from build123d import *

# Parameters (mm, degrees)
SKETCH1_W           = 100
SKETCH1_H           = 48
BOSS_EXTRUDE1_DEPTH = 7
CUT_EXTRUDE1_REACH  = 113.144
SKETCH2_R           = 4
SKETCH2_R_2         = 3.5
SKETCH3_W           = 100
SKETCH3_H           = 8
BOSS_EXTRUDE2_DEPTH = 10.2
SKETCH4_R           = 6.55
CUT_EXTRUDE2_DEPTH  = 5.25
SKETCH5_R           = 2.6
CUT_EXTRUDE3_DEPTH  = 7
SKETCH7_R           = 1.7
CUT_EXTRUDE4_DEPTH  = 112.391382072
CUT_EXTRUDE5_REACH  = 114.249
SKETCH8_R           = 1.7
CUT_EXTRUDE6_DEPTH  = 3
CUT_EXTRUDE7_REACH  = 114.249
SKETCH10_R          = 1.7
CUT_EXTRUDE8_DEPTH  = 3
FILLET1_R           = 20


with BuildPart() as part:
    # Sketch1 → Boss-Extrude1 (new body)
    with BuildSketch(Plane.XY):
        with Locations((50, 24)):
            Rectangle(SKETCH1_W, SKETCH1_H)
    extrude(amount=BOSS_EXTRUDE1_DEPTH)

    # Sketch2 → Cut-Extrude1 (cut, up to next)
    with BuildSketch(Plane.XY.offset(7), mode=Mode.PRIVATE) as cut_extrude1_sk1:
        with BuildLine():
            ThreePointArc((15, 25), (11, 29), (15, 33))
            Line((15, 33), (0, 33))
            Line((0, 33), (0, 25))
            Line((0, 25), (15, 25))
        make_face()
    cut_extrude1_tool1 = extrude(cut_extrude1_sk1.sketch, amount=-CUT_EXTRUDE1_REACH, mode=Mode.PRIVATE) & part.part
    # Sketch2 → Cut-Extrude1 (cut, up to next)
    with BuildSketch(Plane.XY.offset(7), mode=Mode.PRIVATE) as cut_extrude1_sk2:
        with Locations((15, 29)):
            Circle(SKETCH2_R)
    cut_extrude1_tool2 = extrude(cut_extrude1_sk2.sketch, amount=-CUT_EXTRUDE1_REACH, mode=Mode.PRIVATE) & part.part
    # Sketch2 → Cut-Extrude1 (cut, up to next)
    with BuildSketch(Plane.XY.offset(7), mode=Mode.PRIVATE) as cut_extrude1_sk3:
        with Locations((33.75, 29)):
            Circle(SKETCH2_R_2)
    cut_extrude1_tool3 = extrude(cut_extrude1_sk3.sketch, amount=-CUT_EXTRUDE1_REACH, mode=Mode.PRIVATE) & part.part
    # Sketch2 → Cut-Extrude1 (cut, up to next)
    with BuildSketch(Plane.XY.offset(7), mode=Mode.PRIVATE) as cut_extrude1_sk4:
        with Locations((55, 29)):
            Circle(SKETCH2_R_2)
    cut_extrude1_tool4 = extrude(cut_extrude1_sk4.sketch, amount=-CUT_EXTRUDE1_REACH, mode=Mode.PRIVATE) & part.part
    # Sketch2 → Cut-Extrude1 (cut, up to next)
    with BuildSketch(Plane.XY.offset(7), mode=Mode.PRIVATE) as cut_extrude1_sk5:
        with Locations((76.25, 29)):
            Circle(SKETCH2_R_2)
    cut_extrude1_tool5 = extrude(cut_extrude1_sk5.sketch, amount=-CUT_EXTRUDE1_REACH, mode=Mode.PRIVATE) & part.part
    add(cut_extrude1_tool1.solids().sort_by_distance((5.962811, 29, 7))[0], mode=Mode.SUBTRACT)
    add(cut_extrude1_tool2.solids().sort_by_distance((15, 29, 7))[0], mode=Mode.SUBTRACT)
    add(cut_extrude1_tool3.solids().sort_by_distance((33.75, 29, 7))[0], mode=Mode.SUBTRACT)
    add(cut_extrude1_tool4.solids().sort_by_distance((55, 29, 7))[0], mode=Mode.SUBTRACT)
    add(cut_extrude1_tool5.solids().sort_by_distance((76.25, 29, 7))[0], mode=Mode.SUBTRACT)

    # Sketch3 → Boss-Extrude2 (add)
    with BuildSketch(Plane(origin=(0, 0, 0), x_dir=(-1, 0, 0), z_dir=(0, 0, -1))):
        with Locations((-50, 4)):
            Rectangle(SKETCH3_W, SKETCH3_H)
    extrude(amount=BOSS_EXTRUDE2_DEPTH)

    # Sketch4 → Cut-Extrude2 (cut)
    with BuildSketch(Plane(origin=(0, 0, 0), x_dir=(-1, 0, 0), z_dir=(0, 0, -1))):
        with Locations((-76.25, 29)):
            Circle(SKETCH4_R)
        with Locations((-55, 29)):
            Circle(SKETCH4_R)
        with Locations((-33.75, 29)):
            Circle(SKETCH4_R)
    extrude(amount=-CUT_EXTRUDE2_DEPTH, mode=Mode.SUBTRACT)

    # Sketch5 → Cut-Extrude3 (cut)
    with BuildSketch(Plane.XY.offset(7)):
        with Locations((35.000022648, 4.052132501)):
            Circle(SKETCH5_R)
        with Locations((64.999977352, 4)):
            Circle(SKETCH5_R)
    extrude(amount=-CUT_EXTRUDE3_DEPTH, mode=Mode.SUBTRACT)

    # Sketch7 → Cut-Extrude4 (cut, through all)
    with BuildSketch(Plane.XY):
        with Locations((35.000022648, 4.052132501)):
            Circle(SKETCH7_R)
        with Locations((64.999977352, 4)):
            Circle(SKETCH7_R)
    extrude(amount=-CUT_EXTRUDE4_DEPTH, mode=Mode.SUBTRACT)

    # Sketch8 → Cut-Extrude5 (cut, up to next)
    with BuildSketch(Plane.XY.offset(7), mode=Mode.PRIVATE) as cut_extrude5_sk1:
        with Locations((10, 4.052132501)):
            Circle(SKETCH8_R)
    cut_extrude5_tool1 = extrude(cut_extrude5_sk1.sketch, amount=-CUT_EXTRUDE5_REACH, mode=Mode.PRIVATE) & part.part
    # Sketch8 → Cut-Extrude5 (cut, up to next)
    with BuildSketch(Plane.XY.offset(7), mode=Mode.PRIVATE) as cut_extrude5_sk2:
        with Locations((90, 4.052132501)):
            Circle(SKETCH8_R)
    cut_extrude5_tool2 = extrude(cut_extrude5_sk2.sketch, amount=-CUT_EXTRUDE5_REACH, mode=Mode.PRIVATE) & part.part
    add(cut_extrude5_tool1.solids().sort_by_distance((10, 4.052133, 7))[0], mode=Mode.SUBTRACT)
    add(cut_extrude5_tool2.solids().sort_by_distance((90, 4.052133, 7))[0], mode=Mode.SUBTRACT)


with BuildPart() as body_2:
    # Mirror1: mirrored copy
    add(part.part.mirror(Plane.XY.offset(-10.2)))

    # Sketch9 → Cut-Extrude6 (cut)
    with BuildSketch(Plane(origin=(0, 0, -27.4), x_dir=(-1, 0, 0), z_dir=(0, 0, -1))):
        Polygon((-88.267949192, 1.052132501), (-86.535898385, 4.052132501), (-88.267949192, 7.052132501), (-91.732050808, 7.052132501), (-93.464101615, 4.052132501), (-91.732050808, 1.052132501), align=None)
        Polygon((-13.464101615, 4.052132501), (-11.732050808, 1.052132501), (-8.267949192, 1.052132501), (-6.535898385, 4.052132501), (-8.267949192, 7.052132501), (-11.732050808, 7.052132501), align=None)
    extrude(amount=-CUT_EXTRUDE6_DEPTH, mode=Mode.SUBTRACT)

    # Sketch10 → Cut-Extrude7 (cut, up to next)
    with BuildSketch(Plane(origin=(0, 0, -27.4), x_dir=(-1, 0, 0), z_dir=(0, 0, -1)), mode=Mode.PRIVATE) as cut_extrude7_sk1:
        with Locations((-15, 44)):
            Circle(SKETCH10_R)
    cut_extrude7_tool1 = extrude(cut_extrude7_sk1.sketch, amount=-CUT_EXTRUDE7_REACH, mode=Mode.PRIVATE) & body_2.part
    # Sketch10 → Cut-Extrude7 (cut, up to next)
    with BuildSketch(Plane(origin=(0, 0, -27.4), x_dir=(-1, 0, 0), z_dir=(0, 0, -1)), mode=Mode.PRIVATE) as cut_extrude7_sk2:
        with Locations((-15, 14)):
            Circle(SKETCH10_R)
    cut_extrude7_tool2 = extrude(cut_extrude7_sk2.sketch, amount=-CUT_EXTRUDE7_REACH, mode=Mode.PRIVATE) & body_2.part
    add(cut_extrude7_tool1.solids().sort_by_distance((15, 44, -27.4))[0], mode=Mode.SUBTRACT)
    add(cut_extrude7_tool2.solids().sort_by_distance((15, 14, -27.4))[0], mode=Mode.SUBTRACT)

    # Sketch11 → Cut-Extrude8 (cut)
    with BuildSketch(Plane.XY.offset(-20.4)):
        Polygon((18.464101615, 44), (16.732050808, 47), (13.267949192, 47), (11.535898385, 44), (13.267949192, 41), (16.732050808, 41), align=None)
        Polygon((18.464101615, 14), (16.732050808, 17), (13.267949192, 17), (11.535898385, 14), (13.267949192, 11), (16.732050808, 11), align=None)
    extrude(amount=-CUT_EXTRUDE8_DEPTH, mode=Mode.SUBTRACT)

    # Fillet1
    fillet1_edges = [body_2.edges().sort_by_distance(p)[0] for p in [
        (100, 48, -23.9),
    ]]
    fillet(fillet1_edges, radius=FILLET1_R)


solid = body_2.part
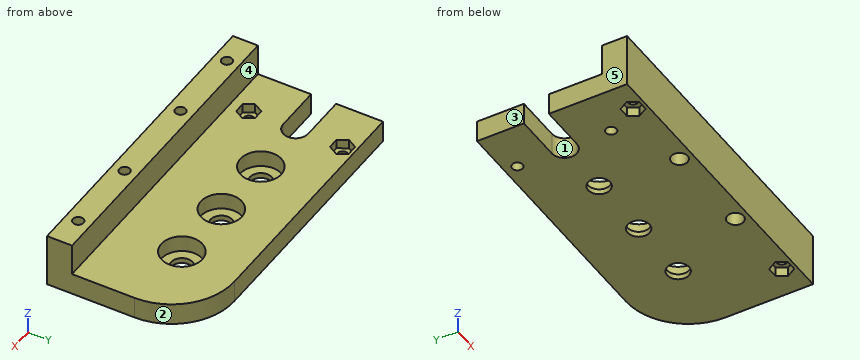
Verification items for the finished model (mm, model axes). Face numbers are marked on the shaded views. A direction names the side the tool comes from. Give positions to 0.01 mm unless a question says otherwise; leave off trailing zeros. Write each loop counter-clockwise with the first axis right and the second up, starting at its lowest first coordinate (ties: lowest second). Pieces come first, ordered by that corner, then holes.
(1) Access from +Z, -Z, +X, -X, +Y, -Y to the whole of each face (thin tool, end or side, straight path). Record for the marked faces 4 and 5.
(2) Cross-section at B-B (x = 76.25). Enter the section's corners in (y, z), plus the area to 3 significant figures.
(3) Material ranges on line 1 (Y direction, x = 15, z = -24.8); line 2 (X direction, y = 5.5, z = -15.25); line 3 (X direction, y = 26, z = -24.5), recorded low to high.
(4) Gauge pin test, flat ends, axial feed: pin 1 (5 mm diameter, centred on x = 69, y = 34, fed in from +Z); pin 2 (3 mm diameter, centred on x = 90, y = 4.05, fed in from +Z); pin 3 (4 mm diameter, centred on x = 79.5, y = 32, fed in from +Z); pin 4 (1.8 mm diameter, centred on x = 11.5, y = 3.5, fed in from -Z). Record the tip position at first contact, or that the pin passes through.
(5) Cross-section at D-D (y = 30). Enter the section's corners in (x, z).
(6) Mould release check, pull along Y, two halves, no side actions. Record for the marked faces 1, 2 and 3: +Y half, -Y half, draft (parallel to the pull), parting line (faces both ways), or undercut.
(7) Cross-section at C-C (z = -14.5). Enter the section's corners in (x, y), plus the area to 3 significant figures.
(8) Cross-section at A-A (x = 10). Enter the section's corners in (y, z).
Worked out:
1. face 4: +Z, +X, -X, +Y
1. face 5: +Z, -Z, -X, +Y, -Y
2. outline: (0, -27.4) - (25.5, -27.4) - (25.5, -25.65) - (22.45, -25.65) - (22.45, -20.4) - (8, -20.4) - (8, -10.2) - (0, -10.2) - close; (32.5, -27.4) - (48, -27.4) - (48, -20.4) - (35.55, -20.4) - (35.55, -25.65) - (32.5, -25.65) - close
2. area: 337 mm2
3. line 1: y = 0 to 12.3, 15.7 to 25, 33 to 42.3, 45.7 to 48
3. line 2: x = 0 to 9.11, 10.89 to 34.11, 35.89 to 64.2, 65.8 to 89.11, 90.89 to 100
3. line 3: x = 17.65 to 27.93, 39.57 to 49.18, 60.82 to 70.43, 82.07 to 100
4. pin 1: stops at z = -20.4
4. pin 2: passes through
4. pin 3: stops at z = -25.65
4. pin 4: stops at z = -24.4
5. outline: (18.87, -27.4) - (30.4, -27.4) - (30.4, -25.65) - (27.28, -25.65) - (27.28, -20.4) - (18.87, -20.4) - close; (37.1, -27.4) - (51.65, -27.4) - (51.65, -25.65) - (48.53, -25.65) - (48.53, -20.4) - (40.22, -20.4) - (40.22, -25.65) - (37.1, -25.65) - close; (58.35, -27.4) - (72.9, -27.4) - (72.9, -25.65) - (69.78, -25.65) - (69.78, -20.4) - (61.47, -20.4) - (61.47, -25.65) - (58.35, -25.65) - close; (79.6, -27.4) - (99.9, -27.4) - (99.9, -20.4) - (82.72, -20.4) - (82.72, -25.65) - (79.6, -25.65) - close
6. face 1: undercut
6. face 2: +Y half
6. face 3: draft
7. outline: (0, 0) - (100, 0) - (100, 8) - (0, 8) - close; hole circle Ø3.4 at (10, 4.05); hole circle Ø3.4 at (35, 4.05); hole circle Ø3.4 at (65, 4); hole circle Ø3.4 at (90, 4.05)
7. area: 764 mm2
8. outline: (0, -27.4) - (1.05, -27.4) - (1.05, -24.4) - (2.35, -24.4) - (2.35, -10.2) - (0, -10.2) - close; (5.75, -24.4) - (7.05, -24.4) - (7.05, -27.4) - (25, -27.4) - (25, -20.4) - (8, -20.4) - (8, -10.2) - (5.75, -10.2) - close; (33, -27.4) - (48, -27.4) - (48, -20.4) - (33, -20.4) - close
